Here's the drawing with two shaded views (mm, measured from the low corner). I have some questions. A direction names the side the tool comes from. Round coordinates to 2 decimals unless told otherwise and drop trailing zeros. Loops run counter-clockwise (first coordinate to the right, second up) from the corner with the lowest first, then second, coordinate; pieces in that order, holes last.
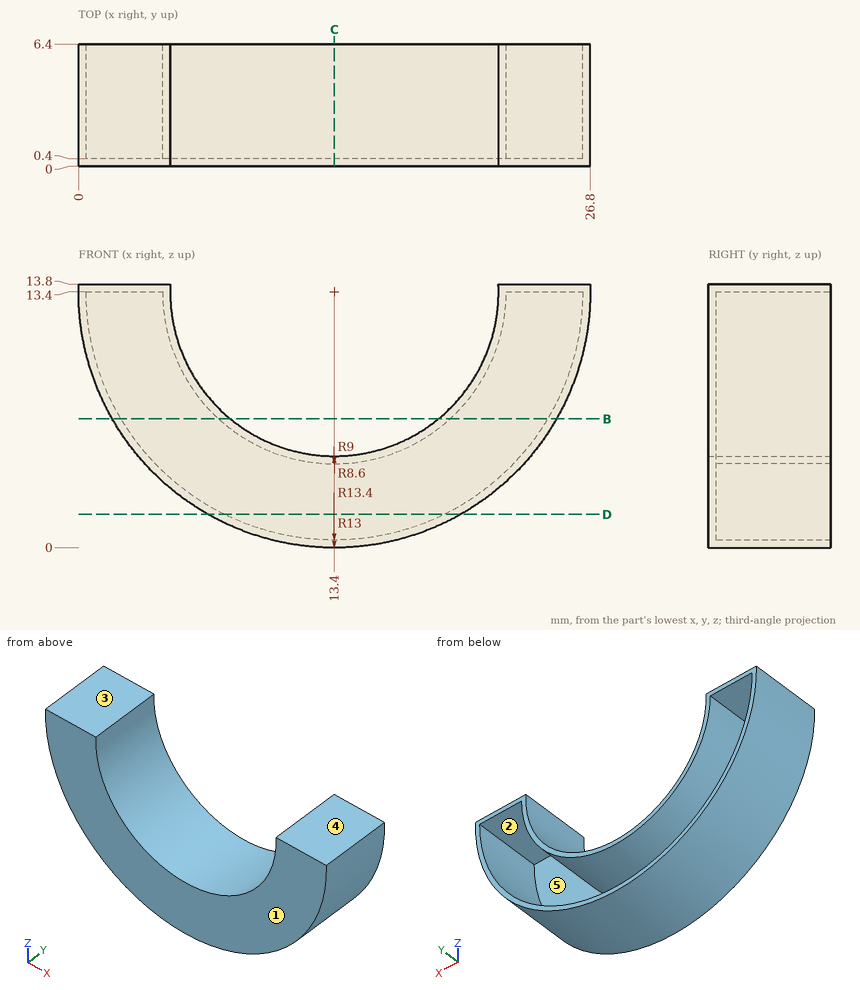
Item 1: If we section it at B-B, the plane z = 6.75: Please give me the cut outline in (x, y).
Results list:
outline: (1.77, 0) - (7.95, 0) - (7.95, 6.4) - (7.34, 6.4) - (7.34, 0.4) - (2.23, 0.4) - (2.23, 6.4) - (1.77, 6.4) - close; (18.85, 0) - (25.03, 0) - (25.03, 6.4) - (24.57, 6.4) - (24.57, 0.4) - (19.46, 0.4) - (19.46, 6.4) - (18.85, 6.4) - close
Item 2: If we section it at D-D, the plane z = 1.75: Please give me the cut outline in (x, y).
Results list:
outline: (6.78, 0) - (20.02, 0) - (20.02, 6.4) - (19.17, 6.4) - (19.17, 0.4) - (7.63, 0.4) - (7.63, 6.4) - (6.78, 6.4) - close
Item 3: If I drill on line 1 along X through (y, z) = (6, 9.5); line 2 along X through (y, z) = (3.25, 11); line 3 along Z through (x, y) = (10.25, 3.75), over which ranges is the centre line in solid material (lowest first)?
Results list:
line 1: x = 0.58 to 1, 5.29 to 5.74, 21.06 to 21.51, 25.8 to 26.22
line 2: x = 0.22 to 0.62, 4.73 to 5.14, 21.66 to 22.07, 26.18 to 26.58
line 3: z = 0.38 to 0.79, 4.97 to 5.4
Item 4: Will these pins go through, and if not, where does the flat tip stop? pin 1 (2 mm diameter, centred on x = 25, y = 4, fed in from -Z); pin 2 (3 mm diameter, centred on x = 14.5, y = 2, fed in from +Z); pin 3 (3 mm diameter, centred on x = 3.5, y = 2, fed in from -Z).
Results list:
pin 1: stops at z = 5.2
pin 2: stops at z = 5.2
pin 3: stops at z = 2.96
Item 5: For the marked faces 4 and 5, which set-ups out of +Z, -Z, +X, -X, +Y, -Y let a thin tool reach every point of the face, with its end or its side?
Results list:
face 4: +Z, +X, -X, +Y, -Y
face 5: +Y
Item 6: If we section it at C-C, the plane x = 13.4: Please give me the cut outline in (y, z).
Results list:
outline: (0, 0) - (6.4, 0) - (6.4, 0.4) - (0.4, 0.4) - (0.4, 4.4) - (6.4, 4.4) - (6.4, 4.8) - (0, 4.8) - close
Item 7: We'd pull the mould along Z, two halves only. Please class the marked faces 1, 2 and 3: released by +Z, released by -Z, zero draft, split by the parting line, or undercut.
Results list:
face 1: zero draft
face 2: undercut
face 3: released by +Z
